from build123d import *

# Parameters (mm, degrees)
F0_W     = 100
F0_H     = 80
F0_R     = 20
F1_DEPTH = 44
F3_DEPTH = 20


with BuildPart() as f1:
    # F0 (on Top) → F1 (new body)
    with BuildSketch(Plane.XY):
        Rectangle(F0_W, F0_H)
        Circle(F0_R, mode=Mode.SUBTRACT)
    extrude(amount=F1_DEPTH)

    # F2 (on face) → F3 (cut)
    with BuildSketch(Plane.XY.offset(44)):
        with BuildLine():
            Line((50, -40), (50, 40))
            Line((50, 40), (-30, 40))
            Line((-30, 40), (-15.1690265486, 13.0345937247))
            ThreePointArc((-15.1690265486, 13.0345937247), (6.9505204492, 18.7534067701), (20, 0))
            ThreePointArc((20, 0), (15.1277749358, -13.0824472287), (2.8849574507, -19.7908317285))
            Line((2.8849574507, -19.7908317285), (14, -40))
            Line((14, -40), (50, -40))
        make_face()
    extrude(amount=-F3_DEPTH, mode=Mode.SUBTRACT)


solid = f1.part
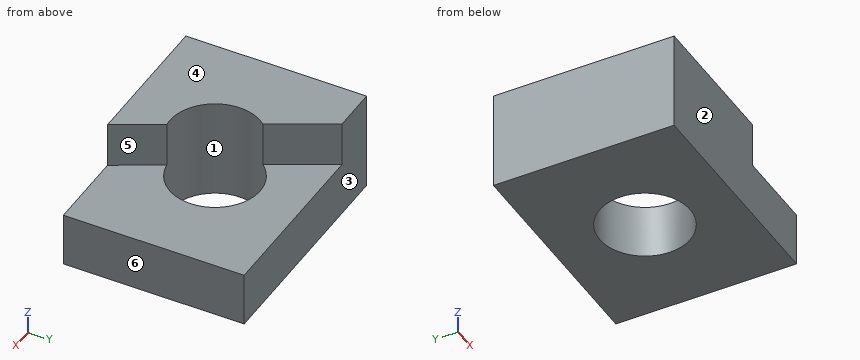
Geometry check sheet. Reference: the model listing, model coordinates, mm. Face numbers are marked on the shaded views. A direction names the side the tool comes from. Coordinates: 2 decimals unless noted, no trailing zeros. Loops run counter-clockwise (first coordinate to the right, second up) from the corner with the lowest first, then second, coordinate; pieces in that order, holes last. Notation, with made-up numbers: (76, -27) - (95, -27) arc R15 ccw to (95, -23) - close; hole circle Ø10 at (-32, 19). An arc over 180 degrees is marked (long way). Use one line per item in the form item = value. Start each with the question number.
Item 1: Section check C-C, the plane z = 21.5. Enter the section's corners in (x, y).
Item 2: Tool access check on the marked faces 5 and 6. Record the directions out of +Z, -Z, +X, -X, +Y, -Y that give a thin tool (end or side, any length) a straight path to the whole face; none if there is none.
Item 3: Section check D-D, the plane z = 39.5. Enter the section's corners in (x, y).
Item 4: Thickness scan on probe 1 along X at (y, z) = (0, 23); probe 2 along Y at (x, z) = (0, 16.5); probe 3 along Y at (x, z) = (0, 35). Record the ranges inside material, lowest first.
Item 5: Section check B-B, the plane y = -14. Enter the section's corners in (x, z), and give its area (3 significant figures).
Item 6: Gauge pin test, flat ends, axial feed: pin 1 (6 mm diameter, centred on x = 11.5, y = 26, fed in from +Z); pin 2 (4 mm diameter, centred on x = -24.5, z = 38, fed in from +Y); pin 3 (5 mm diameter, centred on y = 21.5, z = 25.5, fed in from +X). Record the tip position at first contact, or that the pin passes through.
Item 7: Section check A-A, the plane x = 0. Enter the section's corners in (y, z), and give its area (3 significant figures).
Item 8: Mould release check, pull along Y, two halves, no side actions. Record for the marked faces 1, 2, 3 and 4: +Y half, -Y half, draft (parallel to the pull), parting line (faces both ways), or undercut.
Computed:
q1.outline = (-50, -40) - (50, -40) - (50, 40) - (-50, 40) - close; hole circle Ø40 at (0, 0)
q2.face_5 = +Z, +X, +Y
q2.face_6 = +Z, -Z, +X, +Y, -Y
q3.outline = (-50, -40) - (14, -40) - (2.88, -19.79) arc R20 cw to (-15.17, 13.03) - (-30, 40) - (-50, 40) - close
q4.probe_1 = -50 to -20, 20 to 50
q4.probe_2 = -40 to -20, 20 to 40
q4.probe_3 = -40 to -20
q5.outline = (-50, 0) - (-14.28, 0) - (-14.28, 44) - (-50, 44) - close; (14.28, 0) - (50, 0) - (50, 24) - (14.28, 24) - close
q5.area = 2,430 mm2
q6.pin_1 = 24
q6.pin_2 = 33.64
q6.pin_3 = 50
q7.outline = (-40, 0) - (-20, 0) - (-20, 44) - (-40, 44) - close; (20, 0) - (40, 0) - (40, 24) - (20, 24) - close
q7.area = 1,360 mm2
q8.face_1 = undercut
q8.face_2 = -Y half
q8.face_3 = +Y half
q8.face_4 = draft
